```python
from build123d import *
from build123d.topology import SkipClean

# Parameters (mm, degrees)
SKETCH1_W                           = 47.1
SKETCH1_H                           = 10
BOSS_EXTRUDE1_START                 = 30
BOSS_EXTRUDE1_DEPTH                 = 30
BOSS_EXTRUDE2_START                 = -17.1
SKETCH8_R                           = 18
BOSS_EXTRUDE2_DEPTH                 = 5
M3X0_5_TAPPED_HOLE3_D               = 2.5
M3X0_5_TAPPED_HOLE3_DEPTH           = 10
M3X0_5_TAPPED_HOLE3_TIP             = 0.751075774
M3X0_5_TAPPED_HOLE2_D               = 2.5
M3X0_5_TAPPED_HOLE2_DEPTH           = 5
M3X0_5_TAPPED_HOLE2_TIP             = 0.751075774
M3X0_5_TAPPED_HOLE2_ON_FACE_2_D     = 2.5
M3X0_5_TAPPED_HOLE2_ON_FACE_2_DEPTH = 5
M3X0_5_TAPPED_HOLE2_ON_FACE_2_TIP   = 0.751075774
BOSS_EXTRUDE3_START                 = 5
BOSS_EXTRUDE3_DEPTH                 = 5
TOLERANCING_START                   = 30
TOLERANCING_OUTLINE_R               = 10
TOLERANCING_OUTLINE_R_2             = 9.5
TOLERANCING_DEPTH                   = 52.1
TOLERANCING_2_OUTLINE_R             = 10
TOLERANCING_2_OUTLINE_R_2           = 9.5
TOLERANCING_2_DEPTH                 = 25
TOLERANCING_START_2                 = 47.1
TOLERANCING_3_DEPTH                 = 35


# Read off the part's stored shape, not the designer's step: Tolerancing
with BuildPart() as part:
    # Sketch1 → Revolve1 (revolve)
    with BuildSketch(Plane.XY, mode=Mode.PRIVATE) as revolve1_sk:
        with Locations((23.55, 5)):
            Rectangle(SKETCH1_W, SKETCH1_H)
    revolve(revolve1_sk.sketch.rotate(Axis((0, 0, 0), (1, 0, 0)), 90), axis=Axis((0, 0, 0), (1, 0, 0)))

    # Sketch3 → Boss-Extrude1 (add)
    with BuildSketch(Plane(origin=(47.1, 0, 0), x_dir=(0, 0, -1), z_dir=(1, 0, 0)).offset(BOSS_EXTRUDE1_START)):
        with BuildLine():
            Line((-6.614378278, -7.5), (-6.614378278, 7.5))
            ThreePointArc((-6.614378278, 7.5), (0, 10), (6.614378278, 7.5))
            Line((6.614378278, 7.5), (6.614378278, -7.5))
            ThreePointArc((6.614378278, -7.5), (0, -10), (-6.614378278, -7.5))
        make_face()
    extrude(amount=-BOSS_EXTRUDE1_DEPTH)

    # Sketch8 → Boss-Extrude2 (add)
    with BuildSketch(Plane(origin=(47.1, 0, 0), x_dir=(0, 0, -1), z_dir=(1, 0, 0)).offset(BOSS_EXTRUDE2_START)):
        Circle(SKETCH8_R)
    extrude(amount=-BOSS_EXTRUDE2_DEPTH)

    # M3x0.5 Tapped Hole3
    with Locations(Plane.XY.offset(10)):
        with Locations((20, 0)):
            Hole(M3X0_5_TAPPED_HOLE3_D / 2, depth=M3X0_5_TAPPED_HOLE3_DEPTH)
            with Locations((0, 0, -(M3X0_5_TAPPED_HOLE3_DEPTH + M3X0_5_TAPPED_HOLE3_TIP / 2))):  # 118° drill point
                Cone(0, M3X0_5_TAPPED_HOLE3_D / 2, M3X0_5_TAPPED_HOLE3_TIP, mode=Mode.SUBTRACT)

    # M3x0.5 Tapped Hole2
    with Locations(Plane(origin=(54.6, 0, 6.614378278), x_dir=(1, 0, 0), z_dir=(0, 0, 1))):
        with Locations((0, 0), (15, 0)):
            Hole(M3X0_5_TAPPED_HOLE2_D / 2, depth=M3X0_5_TAPPED_HOLE2_DEPTH)
            with Locations((0, 0, -(M3X0_5_TAPPED_HOLE2_DEPTH + M3X0_5_TAPPED_HOLE2_TIP / 2))):  # 118° drill point
                Cone(0, M3X0_5_TAPPED_HOLE2_D / 2, M3X0_5_TAPPED_HOLE2_TIP, mode=Mode.SUBTRACT)

    # M3x0.5 Tapped Hole2 on face 2
    with Locations(Plane(origin=(69.6, 0, -6.614378278), x_dir=(-1, 0, 0), z_dir=(0, 0, -1))):
        with Locations((0, 0), (15, 0)):
            Hole(M3X0_5_TAPPED_HOLE2_ON_FACE_2_D / 2, depth=M3X0_5_TAPPED_HOLE2_ON_FACE_2_DEPTH)
            with Locations((0, 0, -(M3X0_5_TAPPED_HOLE2_ON_FACE_2_DEPTH + M3X0_5_TAPPED_HOLE2_ON_FACE_2_TIP / 2))):  # 118° drill point
                Cone(0, M3X0_5_TAPPED_HOLE2_ON_FACE_2_D / 2, M3X0_5_TAPPED_HOLE2_ON_FACE_2_TIP, mode=Mode.SUBTRACT)

    # Sketch9 → Boss-Extrude3 (add)
    with SkipClean():  # the faces are left unmerged after this step: merging them gives an invalid solid
        with BuildSketch(Plane(origin=(77.1, 0, 0), x_dir=(0, 0, -1), z_dir=(1, 0, 0)).offset(BOSS_EXTRUDE3_START)):
            with BuildLine():
                Line((6.614378278, -7.5), (6.614378278, 7.5))
                ThreePointArc((6.614378278, 7.5), (0, 10), (-6.614378278, 7.5))
                Line((-6.614378278, 7.5), (-6.614378278, -7.5))
                ThreePointArc((-6.614378278, -7.5), (0, -10), (6.614378278, -7.5))
            make_face()
        extrude(amount=-BOSS_EXTRUDE3_DEPTH)

    # Tolerancing outline → Tolerancing (cut)
    with BuildSketch(Plane.YZ.offset(TOLERANCING_START)):
        Circle(TOLERANCING_OUTLINE_R)
        Circle(TOLERANCING_OUTLINE_R_2, mode=Mode.SUBTRACT)
    extrude(amount=TOLERANCING_DEPTH, mode=Mode.SUBTRACT)

    # Tolerancing 2 outline → Tolerancing 2 (cut)
    with BuildSketch(Plane.YZ):
        Circle(TOLERANCING_2_OUTLINE_R)
        Circle(TOLERANCING_2_OUTLINE_R_2, mode=Mode.SUBTRACT)
    extrude(amount=TOLERANCING_2_DEPTH, mode=Mode.SUBTRACT)

    # Tolerancing 3 outline → Tolerancing 3 (cut)
    with BuildSketch(Plane.YZ.offset(TOLERANCING_START_2)):
        with BuildLine():
            Line((-7.270789385, 6.114378278), (7.270789385, 6.114378278))
            ThreePointArc((7.270789385, 6.114378278), (7.049374529, 6.368384313), (6.819090848, 6.614378278))
            Line((6.819090848, 6.614378278), (-6.819090848, 6.614378278))
            ThreePointArc((-6.819090848, 6.614378278), (-7.049374529, 6.368384313), (-7.270789385, 6.114378278))
        make_face()
        with BuildLine():
            ThreePointArc((6.819090848, -6.614378278), (7.049374529, -6.368384313), (7.270789385, -6.114378278))
            Line((7.270789385, -6.114378278), (-7.270789385, -6.114378278))
            ThreePointArc((-7.270789385, -6.114378278), (-7.049374529, -6.368384313), (-6.819090848, -6.614378278))
            Line((-6.819090848, -6.614378278), (6.819090848, -6.614378278))
        make_face()
    extrude(amount=TOLERANCING_3_DEPTH, mode=Mode.SUBTRACT)


solid = part.part
```
Design review of the part built by this model. Coordinates are the model's own, in mm. A direction names the side the tool comes from. Coordinates: 2 decimals unless noted, no trailing zeros. Order: outer loops, then holes, each group sorted by start corner. A loop starts at its lowest first (then second) coordinate and runs counter-clockwise, first axis right, second up.
1) Take a section at D-D, the plane z = -8.5. Give the boundary of the cut face in (x, y).
2) Mouldability with a two-part tool opening along X and no side actions: class faces 1 (the flat face through (82.1, 0, 0)), 2 (the conical face through (69.817, 0.01, -0.994)), 3 (the cylindrical face through (27.535, 17.847, 2.343)), 4 (the flat face through (0, 0, 0)) as +X half, -X half, draft (parallel to the pull), parting line (faces both ways), or undercut.
3) Take a section at C-C, the plane x = 77.5. Give the boundary of the cut face in (y, z).
4) Take a section at A-A, the plane z = -4. Give the boundary of the cut face in (x, y), and give its area (3 significant figures).
5) For faces 5 (the flat face through (64, 0, -6.114)), 6 (the cylindrical face through (70.85, 0.05, 3.83)), 7 (the cylindrical face through (49.896, 8.776, -3.639)), 8 (the cylindrical face through (70.755, -0.479, -3.833)), 9 (the flat face through (64, 0, 6.114)), list the 3-axis set-ups (+Z, -Z, +X, -X, +Y, -Y) from which the entire face can be reached by the end or side of a thin tool; tool diameter is ignored.
6) Wall thickness on line 1 along X through (y, z) = (0, 4); line 2 along X through (y, z) = (0, -3.4); line 3 along X through (y, z) = (-11, -1): over which ranges is each line inside the solid? List them lowest first.
7) Clearance check with flat-ended pins moving along their axes: pin 1 (2 mm diameter, centred on x = 69.6, y = 0, fed in from -Z); pin 2 (10 mm diameter, centred on x = 70.5, y = 11, fed in from +Z); pin 3 (4.5 mm diameter, centred on x = 62.5, y = 3.5, fed in from -Z); pin 4 (1 mm diameter, centred on x = 60, y = 10.5, fed in from -Z). State where each tip first meets the part, or that it passes through.
8) Take a section at B-B, the plane y = 2.5. Give the boundary of the cut face in (x, z), and give its area (3 significant figures).
Returned:
1. outline: (0, -4.24) - (25, -4.24) - (25, -15.87) - (30, -15.87) - (30, -4.24) - (47.1, -4.24) - (47.1, 4.24) - (30, 4.24) - (30, 15.87) - (25, 15.87) - (25, 4.24) - (0, 4.24) - close
2. face 1: +X half
2. face 2: undercut
2. face 3: draft
2. face 4: -X half
3. outline: (-7.27, -6.11) - (7.27, -6.11) arc R9.5 ccw to (7.27, 6.11) - (-7.27, 6.11) arc R9.5 ccw to start
4. outline: (0, -8.62) - (25, -8.62) - (25, -17.55) - (30, -17.55) - (30, -8.62) - (82.1, -8.62) - (82.1, 8.62) - (30, 8.62) - (30, 17.55) - (25, 17.55) - (25, 8.62) - (0, 8.62) - close; hole circle Ø2.5 at (54.6, 0); hole circle Ø2.5 at (69.6, 0)
4. area: 1,490 mm2
5. face 5: -Z, +X, +Y, -Y
5. face 6: +Z
5. face 7: +X
5. face 8: -Z
5. face 9: +Z, +X, +Y, -Y
6. line 1: x = 0 to 18.75, 21.25 to 53.35, 55.85 to 68.35, 70.85 to 82.1
6. line 2: x = 0 to 53.35, 55.85 to 68.35, 70.85 to 82.1
6. line 3: x = 25 to 30
7. pin 1: stops at z = -1.46
7. pin 2: stops at z = 6.11
7. pin 3: stops at z = -6.11
7. pin 4: passes through
8. outline: (0, -9.17) - (25, -9.17) - (25, -17.83) - (30, -17.83) - (30, -9.17) - (47.1, -9.17) - (47.1, -6.11) - (82.1, -6.11) - (82.1, 6.11) - (47.1, 6.11) - (47.1, 9.17) - (30, 9.17) - (30, 17.83) - (25, 17.83) - (25, 9.17) - (0, 9.17) - close
8. area: 1,380 mm2
